Could you check a few things on this model? Use its own coordinates, in mm. A direction names the side the tool comes from. Give positions to 0.01 mm unless a question says otherwise; leave off trailing zeros. Order: outer loops, then holes, each group sorted by start corner. A loop starts at its lowest first (then second) coordinate and runs counter-clockwise, first axis right, second up. Notation, with made-up numbers: (-4.75, 12.5) -> (4.25, 12.5) arc R15 cw to (4.25, 21.5) -> close; hole circle Ø10 at (-1, -22). An arc over 180 degrees is marked (long way). Answer as CSV lines item,"result". Start each with the question number.
(1) Will these pins go through, and if not, where does the flat tip stop? pin 1 Ø3 at (x, y) = (2.5, 9) entering from +Z; pin 2 Ø1 at (x, y) = (1.5, 6) entering from -Z; pin 3 Ø7.5 at (x, z) = (11, -11) entering from +Y.
(2) We'd pull the mould along Z, two halves only. Please class faces 3 (the face through (9.1, 10.9, 0)), 4 (the face through (9.1, 1.5, -10.9)), 5 (the face through (9.6, 0.74, -12.59)): released by +Z, released by -Z, zero draft, split by the parting line, or undercut.
(3) I want a section at A-A (y = 12.5). Please give me the cut outline in (x, z).
(4) I want a section at C-C (x = 7.5). Please give me the cut outline in (y, z), plus the area to 3 significant figures.
(5) I need wall thicknesses on L1, parallel to X at y = 0.5, z = -12.5; L2, parallel to Z at x = 3, y = 11.5; L3, parallel to Y at x = 7.5, z = -0.85. Which ranges of each line are inside material? Lowest first, please.
(6) I want a section at B-B (z = -12.5). Please give me the cut outline in (x, y), plus the area to 3 significant figures.
(7) On a 3-axis mill with a long thin cutter (end or side, diameter ignored), from which of +Z, -Z, +X, -X, +Y, -Y can I reach the whole of each face in a straight line? I mean faces 1 (the face through (7, 20, -1)), 2 (the face through (9.1, 10.6, -1.5)). Say none if no direction works.
(8) I want a section at D-D (x = 11). Please give me the cut outline in (y, z).
```python
from build123d import *

# Parameters (mm, degrees)
EXTRUDE_THIN1_DEPTH        = 15
F_4_2_4_2_DIAMETER_HOLE1_D = 4.2
F_4_2_4_2_DIAMETER_HOLE2_D = 4.2
FILLET1_R                  = 1.5


with BuildPart() as part:
    # Sketch1 → Extrude-Thin1 (new body)
    with BuildSketch(Plane(origin=(0, 0, 0), x_dir=(0, 0, -1), z_dir=(1, 0, 0))):
        with BuildLine():
            Line((0, 20), (0, 1.5))
            ThreePointArc((0, 1.5), (0.439339828, 0.439339828), (1.5, 0))
            Line((1.5, 0), (20, 0))
            Line((20, 0), (20, 1.5))
            Line((20, 1.5), (1.5, 1.5))
            Line((1.5, 1.5), (1.5, 20))
            Line((1.5, 20), (0, 20))
        make_face()
    extrude(amount=EXTRUDE_THIN1_DEPTH)

    # Ø4.2 (4.2) Diameter Hole1 (through all)
    with Locations(Plane(origin=(0, 1.5, 0), x_dir=(1, 0, 0), z_dir=(0, 1, 0))):
        with Locations((7.5, 12.5)):
            Hole(F_4_2_4_2_DIAMETER_HOLE1_D / 2)

    # Ø4.2 (4.2) Diameter Hole2 (through all)
    with Locations(Plane(origin=(0, 0, -1.5), x_dir=(-1, 0, 0), z_dir=(0, 0, -1))):
        with Locations((-7.5, 12.5)):
            Hole(F_4_2_4_2_DIAMETER_HOLE2_D / 2)

    # Fillet1
    fillet1_edges = [part.edges().sort_by_distance(p)[0] for p in [
        (15, 20, -0.75),
        (0, 20, -0.75),
        (15, 0.75, -20),
        (0, 0.75, -20),
    ]]
    fillet(fillet1_edges, radius=FILLET1_R)


solid = part.part
```
Final values:
1,pin 1,"z = 0"
1,pin 2,"z = -1.5"
1,pin 3,"y = 1.5"
2,face 3,"released by +Z"
2,face 4,"zero draft"
2,face 5,"undercut"
3,outline,"(0, -1.5) -> (5.4, -1.5) -> (5.4, 0) -> (0, 0) -> close; (9.6, -1.5) -> (15, -1.5) -> (15, 0) -> (9.6, 0) -> close"
4,outline,"(0, -20) -> (1.5, -20) -> (1.5, -14.6) -> (0, -14.6) -> close; (0, -10.4) -> (1.5, -10.4) -> (1.5, -1.5) -> (10.4, -1.5) -> (10.4, 0) -> (1.5, 0) arc R1.5 ccw to (0, -1.5) -> close; (14.6, -1.5) -> (20, -1.5) -> (20, 0) -> (14.6, 0) -> close"
4,area,"44.7 mm²"
5,L1,"0 to 5.4, 9.6 to 15"
5,L2,"-1.5 to 0"
5,L3,"0.15 to 10.4, 14.6 to 20"
6,outline,"(0, 0) -> (5.4, 0) -> (5.4, 1.5) -> (0, 1.5) -> close; (9.6, 0) -> (15, 0) -> (15, 1.5) -> (9.6, 1.5) -> close"
6,area,"16.2 mm²"
7,face 1,"+Z, -Z, +X, -X, +Y"
7,face 2,"-Z, +X, -X, +Y"
8,outline,"(0, -20) -> (1.5, -20) -> (1.5, -1.5) -> (20, -1.5) -> (20, 0) -> (1.5, 0) arc R1.5 ccw to (0, -1.5) -> close"
